```python
from build123d import *


with BuildPart() as part:
    # Sketch2 → Revolve1 (revolve)
    with BuildSketch(Plane.XY):
        Polygon((5.5, 0), (5.5, 4), (4.5, 4), (3.5, 5), (0.5, 5), (0.5, 8), (0, 8), (0, 5), (-2, 5), (-2, 0), align=None)
    revolve(axis=Axis((-2, 0, 0), (1, 0, 0)))

    # Sketch4 → Revolve2 (revolve)
    with BuildSketch(Plane.XY):
        with BuildLine():
            Line((0, 4.5), (-3, 4.5))
            Line((-3, 4.5), (-14.879552076, 9.282911506))
            ThreePointArc((-14.879552076, 9.282911506), (-17.339156162, 9.184522448), (-18.897161062, 7.278753994))
            ThreePointArc((-18.897161062, 7.278753994), (-19.617023423, 3.670972882), (-19.858362338, 0))
            Line((-19.858362338, 0), (0, 0))
            Line((0, 0), (0, 4.5))
        make_face()
    revolve(axis=Axis((0, 0, 0), (-1, 0, 0)))


solid = part.part
```
Part model, mm, in its own coordinate system. A direction names the side the tool comes from. Round coordinates to 2 decimals unless told otherwise and drop trailing zeros. Order: outer loops, then holes, each group sorted by start corner. A loop starts at its lowest first (then second) coordinate and runs counter-clockwise, first axis right, second up. Notation, with made-up numbers: M 31,35.5 L 71,35.5 A21 ccw 71,66.5 Z; hole C 61.25,62 d1. An arc over 180 degrees is marked long. Put each result on its own line as item: value. Start each with the question number.
1. Slice it at A-A on y = 0. List the corners of the cut face in (x, z).
2. Tool access for faces 4 (the face through (-2.51, -0.59, -4.46)), 5 (the face through (1.98, -1.08, -4.88)), 6 (the face through (5.5, 0, 0)): list every direction of +Z, -Z, +X, -X, +Y, -Y with a clear straight run to the whole face (end or side of a thin tool).
3. Two-plate mould, pull along X, no slides. Class faces 1 (the face through (4.993, -0.867, -3.905)), 2 (the face through (0, -0.1, -5.2)), 3 (the face through (0.5, 0.1, -5.2)): +X half, -X half, draft (parallel to the pull), parting line (faces both ways), or undercut.
4. Slice it at D-D on x = -6. List the corners of the cut face in (y, z).
5. Drop flat-ended pins along their axis: pin 1 (8 mm diameter, centred on x = -3, z = 2.5, fed in from +Y); pin 2 (2 mm diameter, centred on x = -15, z = -6, fed in from -Y); pin 3 (5 mm diameter, centred on x = -12.5, y = -5.5, fed in from +Z). Give the stop position or say it passes through.
6. Slice it at C-C on x = -11.5. List the corners of the cut face in (y, z), then the cut area to 3 significant figures.
7. Drill centre lines: probe 1 along X at (y, z) = (0.5, 0.25); probe 2 along X at (y, z) = (4, -5); probe 3 along X at (y, z) = (4.5, -6.5). Where is each one in solid material? Low to high. Write a range as [from, to].
Findings:
1. outline: M -18.9,-7.28 A3 ccw -14.88,-9.28 L -3,-4.5 L -2,-4.5 L -2,-5 L 0,-5 L 0,-8 L 0.5,-8 L 0.5,-5 L 3.5,-5 L 4.5,-4 L 5.5,-4 L 5.5,4 L 4.5,4 L 3.5,5 L 0.5,5 L 0.5,8 L 0,8 L 0,5 L -2,5 L -2,4.5 L -3,4.5 L -14.88,9.28 A3 ccw -18.9,7.28 A28.04 ccw Z
2. face 4: none
2. face 5: +X
2. face 6: +Z, -Z, +X, +Y, -Y
3. face 1: draft
3. face 2: undercut
3. face 3: +X half
4. outline: C 0,0 d11.42
5. pin 1: y = 8
5. pin 2: y = -7.95
5. pin 3: z = 8.23
6. outline: C 0,0 d15.84
6. area: 197 mm2
7. probe 1: [-19.85, 5.5]
7. probe 2: [-19.12, -7.73], [0, 0.5]
7. probe 3: [-18.65, -11.46], [0, 0.5]
